Input: part model. Units: mm. Frame: model coordinates. A direction names the side the tool comes from. Coordinates: 2 decimals unless noted, no trailing zeros. Order: outer loops, then holes, each group sorted by start corner. A loop starts at its lowest first (then second) coordinate and runs counter-clockwise, first axis right, second up. Notation, with made-up numbers: (69.5, 43.5) - (119.5, 43.5) arc R25 cw to (119.5, 69.5) - close; hole circle Ø1 at (89.5, -9). An arc over 180 degrees is marked (long way). Use a Markdown table: item, result. Add a question column.
Autodesk Inventor part; units mm, degrees
ref_plane "YZ Plane" through (0, 0, 0) normal (1, 0, 0) x (0, 1, 0)
ref_plane "XZ Plane" through (0, 0, 0) normal (0, 1, 0) x (-1, 0, 0)
ref_plane "XY Plane" through (0, 0, 0) normal (0, 0, 1) x (1, 0, 0)
sketch "Sketch1" plane through (0, 0, 0) normal (0, 1, 0) x (-1, 0, 0)
  circle A0 centre (0, 0) radius 51.45
  circle A1 centre (0, 0) radius 2
  line L0 (4, -3) -> (43.45, -3)
  line L1 (0.5981, 4.9641) -> (-19.1269, 39.1288)
  line L2 (-4.5981, -1.9641) -> (-24.3231, -36.1288)
  line L3 (4, 3) -> (43.45, 3)
  line L4 (-4.5981, 1.9641) -> (-24.3231, 36.1288)
  line L5 (0.5981, -4.9641) -> (-19.1269, -39.1288)
  arc A2 (4, 3) -> (0.5981, 4.9641) centre (0, 0) ccw
  arc A3 (-4.5981, 1.9641) -> (-4.5981, -1.9641) centre (0, 0) ccw
  arc A4 (0.5981, -4.9641) -> (4, -3) centre (0, 0) ccw
  arc A5 (-23.2687, 34.3026) -> (-23.2687, -34.3026) centre (0, 0) ccw
  arc A6 (-18.0726, -37.3026) -> (41.3413, -3) centre (0, 0) ccw
  arc A7 (41.3413, 3) -> (-18.0726, 37.3026) centre (0, 0) ccw
  circle A8 centre (-23.127, -40.341) radius 4
  circle A9 centre (23.3728, -40.199) radius 4
  circle A10 centre (46.4998, 0.1419) radius 4
  circle A11 centre (23.127, 40.341) radius 4
  circle A12 centre (-23.3728, 40.199) radius 4
  circle A13 centre (-46.4998, -0.1419) radius 4
  dimension "d0" = 102.9
  dimension "d2" = 4
  dimension "d7" = 360
  dimension "d9" = 6
  dimension "d12" = 360
  dimension "d16" = 8
  dimension "d17" = 46.5
  dimension "d20" = 360
extrude "Extrusion2" add sketch "Sketch1" along normal blind 6
properties part number "reaction wheel" material "PC/ABS Plastic"
1) Contact query for flat-ended pins moving along their axis: P1, Ø2.5, axis at x = 0, z = 0, coming from the +Y side; P2, Ø3, axis at x = -31, y = 1.5, coming from the -Z side; P3, Ø2, axis at x = 39.5, y = 5.5, coming from the -Z side. Output: stop coordinate, or through.
2) Pull-direction query (Z, two-part tool) for faces 1 (the cylindrical face through (37.921, 2.958, -34.772)), 2 (the cylindrical face through (0, 3, 2)), 3 (the flat face through (0, 0, -4)); classes: pulls with the +Z half, pulls with the -Z half, needs draft (parallel to the pull), parting line crosses it, or undercut.
3) Material intervals for L1, parallel to X at y = 4.25, z = 6; L2, parallel to Z at x = 21, y = 4.65; L3, parallel to X at y = 4.2, z = -22.5, sorted ascending.
4) Cut plane B-B (x = -6.5). Return the cut outline in (y, z), and give its area (3 significant figures).
5) Reachability of faces 4 (the flat face through (0, 6, -4)), 5 (the flat face through (-22, 3, 3)) from +Z, -Z, +X, -X, +Y, -Y: full face, straight path, thin tool, end or side. Return the list, or none.
6) Cut plane C-C (y = 1.9). State how many separate pieces and enclosed holes the cut face has, and give its area (3 significant figures).
7) Cut plane D-D (z = 13). Return the cut outline in (x, y).
8) Cut plane A-A (x = 29). Return the cut outline in (y, z), and give its area (3 significant figures).
Computed:
| question | item | result |
|---|---|---|
| 1 | P1 | passes through |
| 1 | P2 | stops at z = -42.15 |
| 1 | P3 | stops at z = -34.13 |
| 2 | face 1 | parting line crosses it |
| 2 | face 2 | undercut |
| 2 | face 3 | needs draft |
| 3 | L1 | x = -51.1 to -41.01, 0 to 6.93, 41.01 to 51.1 |
| 3 | L2 | z = -46.97 to -43.73, -36.95 to -30.37, 30.37 to 36.98, 43.42 to 46.97 |
| 3 | L3 | x = -46.27 to -34.81, 9.53 to 16.45, 34.81 to 46.27 |
| 4 | outline | (0, -51.04) - (6, -51.04) - (6, -40.94) - (0, -40.94) - close; (0, -3) - (6, -3) - (6, 3) - (0, 3) - close; (0, 40.94) - (6, 40.94) - (6, 51.04) - (0, 51.04) - close |
| 4 | area | 157 mm2 |
| 5 | face 4 | +Z, -Z, +X, -X, +Y |
| 5 | face 5 | +Y, -Y |
| 6 | separate pieces | 1 |
| 6 | enclosed holes | 10 |
| 6 | area | 3,340 mm2 |
| 7 | outline | (-49.78, 0) - (-39.36, 0) - (-39.36, 6) - (-49.78, 6) - close; (4.04, 0) - (10.97, 0) - (10.97, 6) - (4.04, 6) - close; (39.36, 0) - (49.78, 0) - (49.78, 6) - (39.36, 6) - close |
| 8 | outline | (0, -42.5) - (6, -42.5) - (6, -29.62) - (0, -29.62) - close; (0, 29.62) - (6, 29.62) - (6, 42.5) - (0, 42.5) - close |
| 8 | area | 155 mm2 |
